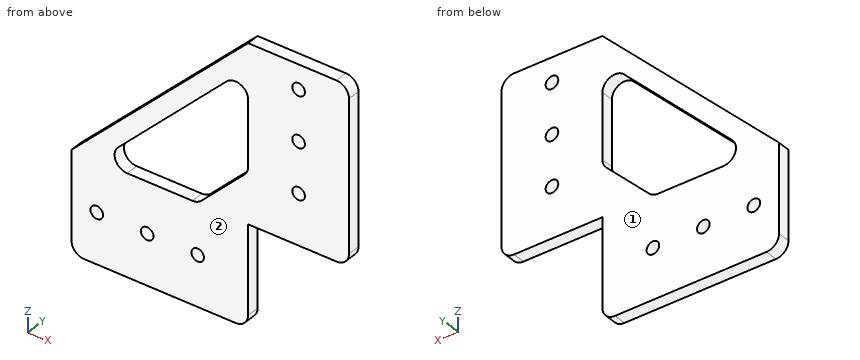
Autodesk Inventor part; units mm, degrees
ref_plane "YZ Plane" through (0, 0, 0) normal (1, 0, 0) x (0, 1, 0)
ref_plane "XZ Plane" through (0, 0, 0) normal (0, 1, 0) x (-1, 0, 0)
ref_plane "XY Plane" through (0, 0, 0) normal (0, 0, 1) x (1, 0, 0)
sketch "Sketch1" plane through (0, 0, 0) normal (0, 1, 0) x (-1, 0, 0)
  line L0 (28.575, 5.149) -> (50.5384, 5.149)
  line L1 (0, 33.724) -> (0, 50.8)
  line L2 (25.4, 8.324) -> (25.4, 30.549)
  line L3 (25.4, 30.549) -> (3.175, 30.549)
  arc A0 (25.4, 8.324) -> (28.575, 5.149) centre (28.575, 8.324) ccw
  arc A1 (0, 33.724) -> (3.175, 30.549) centre (3.175, 33.724) ccw
  circle A2 centre (12.7, 43.249) radius 1.5875
  circle A3 centre (38.1, 17.849) radius 1.5875
  circle A4 centre (50.8, 17.849) radius 1.5875
  circle A5 centre (63.5, 17.849) radius 1.5875
  line L4 (50.5384, 5.149) -> (66.675, 5.149)
  line L5 (69.85, 8.324) -> (69.85, 30.549)
  arc A6 (66.675, 5.149) -> (69.85, 8.324) centre (66.675, 8.324) ccw
  circle A7 centre (12.7, 55.949) radius 1.5875
  circle A8 centre (12.7, 68.649) radius 1.5875
  line L6 (0, 50.8) -> (0, 71.6223)
  line L7 (3.175, 74.7973) -> (25.4, 74.7973)
  arc A9 (3.175, 74.7973) -> (0, 71.6223) centre (3.175, 71.6223) ccw
  line L8 (25.4, 74.7973) -> (69.85, 30.549)
  line L9 (26.3299, 42.319) -> (37.1701, 31.4789)
  line L10 (39.4151, 30.549) -> (55.8349, 30.549)
  line L11 (58.0799, 35.969) -> (30.8201, 63.2289)
  line L12 (25.4, 60.9838) -> (25.4, 44.5641)
  arc A10 (30.8201, 63.2289) -> (25.4, 60.9838) centre (28.575, 60.9838) ccw
  arc A11 (55.8349, 30.549) -> (58.0799, 35.969) centre (55.8349, 33.724) ccw
  arc A12 (37.1701, 31.4789) -> (39.4151, 30.549) centre (39.4151, 33.724) ccw
  arc A13 (25.4, 44.5641) -> (26.3299, 42.319) centre (28.575, 44.5641) ccw
  point P0 (0, 0)
  point P1 (25.4, 5.149)
  point P2 (0, 42.262)
  point P3 (25.4, 19.4365)
  point P4 (39.5567, 5.149)
  point P5 (69.85, 5.149)
  point P6 (0, 74.7973)
  point P7 (14.2875, 74.7973)
  point P8 (38.1, 30.549)
  point P9 (63.5, 30.549)
  dimension "d0" = 50.8
  dimension "d1" = 50.8
  dimension "d2" = 25.4
  dimension "d3" = 3.175
  dimension "d4" = 3.175
  dimension "d5" = 12.7
  dimension "d6" = 12.7
  dimension "d7" = 3.175
  dimension "d8" = 12.7
  dimension "d9" = 12.7
  dimension "d12" = 12.7
  dimension "d17" = 25.4
  dimension "d18" = 6.35
  dimension "d19" = 3.175
  dimension "d22" = 12.7
  dimension "d27" = 25.4
  dimension "d28" = 6.35
  dimension "d29" = 3.175
  dimension "d30" = 25.4
  dimension "d31" = 6.35
  dimension "d32" = 3.175
extrude "Extrusion1" add sketch "Sketch1" along normal blind 3.175
properties part number "Cut L-Bracket (5x5)"
Verification items for the finished model (mm, model axes). Face numbers are marked on the shaded views. Coordinates: 2 decimals unless noted, no trailing zeros. Loops run counter-clockwise (first coordinate to the right, second up) from the corner with the lowest first, then second, coordinate; pieces in that order, holes last. Notation, with made-up numbers: M 88.5,77.25 L 100.5,77.25 A7 cw 100.5,81.25 Z; hole C 76.5,-15.5 d2. An arc over 180 degrees is marked long. One line per item, written item: value.
1. Mould release check, pull along Y, two halves, no side actions. Record for the marked faces 1 and 2: pulls with the +Y half, pulls with the -Y half, needs draft (parallel to the pull), parting line crosses it, or undercut.
Answers follow:
face 1: pulls with the +Y half
face 2: pulls with the -Y half
2. Material ranges on line 1 along Z through (x, y) = (-12.7, 1.75); line 2 along X through (y, z) = (0.3, 44.5); line 3 along Z through (x, y) = (-38.1, 1), recorded low to high. Write a range as from..to.
Answers follow:
line 1: 30.55..41.66, 44.84..54.36, 57.54..67.06, 70.24..74.8
line 2: -55.84..-49.55, -25.4..-13.68, -11.72..0
line 3: 5.15..16.26, 19.44..30.83, 55.95..62.15
3. Section check D-D on y = 0.7. Give the number of separate pieces and of enclosed holes in the cut face, plus the area to 3 significant figures.
Answers follow:
separate pieces: 1
enclosed holes: 7
area: 2,560 mm^2
4. Section check B-B on z = 51.5. Record the cut outline in (x, y) (1 decimal).
Answers follow:
outline: M -48.8,0 L -42.5,0 L -42.5,3.2 L -48.8,3.2 Z; M -25.4,0 L 0,0 L 0,3.2 L -25.4,3.2 Z
5. Section check A-A on x = -12.7. Record the cut outline in (y, z) (1 decimal), plus the area to 3 significant figures.
Answers follow:
outline: M 0,30.5 L 3.2,30.5 L 3.2,41.7 L 0,41.7 Z; M 0,44.8 L 3.2,44.8 L 3.2,54.4 L 0,54.4 Z; M 0,57.5 L 3.2,57.5 L 3.2,67.1 L 0,67.1 Z; M 0,70.2 L 3.2,70.2 L 3.2,74.8 L 0,74.8 Z
area: 110 mm^2
6. Gauge pin test, flat ends, axial feed: P1, Ø1, axis at y = 1.5, z = 49.5, coming from the -X side; P2, Ø1, axis at x = -20.5, y = 0.5, coming from the -Z side. Record the tip position at first contact, or that the pin passes through.
Answers follow:
P1: x = -51.31
P2: z = 30.55
7. Section check C-C on x = -63.5. Record the cut outline in (y, z) (1 decimal).
Answers follow:
outline: M 0,5.1 L 3.2,5.1 L 3.2,16.3 L 0,16.3 Z; M 0,19.4 L 3.2,19.4 L 3.2,36.9 L 0,36.9 Z
